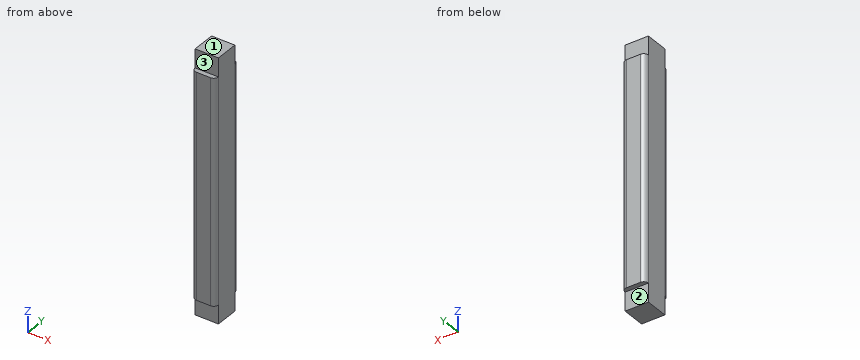
```python
from build123d import *

# Parameters (mm, degrees)
ESQUISSE1_W             = 25
ESQUISSE1_H             = 35
BOSS_EXTRU_1_DEPTH      = 280
ESQUISSE2_OUTSIDE_W     = 83.656
ESQUISSE2_OUTSIDE_H     = 93.656
ESQUISSE2_OUTSIDE_W_2   = 25
ESQUISSE2_OUTSIDE_H_2   = 25
ENL_V_MAT_EXTRU_2_DEPTH = 20
ENL_V_START             = -280
ESQUISSE2_2_OUTSIDE_W   = 83.656
ESQUISSE2_2_OUTSIDE_H   = 93.656
ESQUISSE2_2_OUTSIDE_W_2 = 25
ESQUISSE2_2_OUTSIDE_H_2 = 25
ENL_V_MAT_EXTRU_3_DEPTH = 20
CONG_1_R                = 5


with BuildPart() as part:
    # Esquisse1 → Boss.-Extru.1 (new body)
    with BuildSketch(Plane.XY):
        with Locations((12.5, 17.5)):
            Rectangle(ESQUISSE1_W, ESQUISSE1_H)
    extrude(amount=BOSS_EXTRU_1_DEPTH)

    # Esquisse2 outside → Enlèv. mat.-Extru.2 (cut)
    with BuildSketch(Plane.XY.offset(280)):
        with Locations((12.5, 17.5)):
            Rectangle(ESQUISSE2_OUTSIDE_W, ESQUISSE2_OUTSIDE_H)
        with Locations((12.5, 17.5)):
            Rectangle(ESQUISSE2_OUTSIDE_W_2, ESQUISSE2_OUTSIDE_H_2, mode=Mode.SUBTRACT)
    extrude(amount=-ENL_V_MAT_EXTRU_2_DEPTH, mode=Mode.SUBTRACT)

    # Esquisse2<2> outside → Enlèv. mat.-Extru.3 (cut)
    with BuildSketch(Plane.XY.offset(280).offset(ENL_V_START)):
        with Locations((12.5, 17.5)):
            Rectangle(ESQUISSE2_2_OUTSIDE_W, ESQUISSE2_2_OUTSIDE_H)
        with Locations((12.5, 17.5)):
            Rectangle(ESQUISSE2_2_OUTSIDE_W_2, ESQUISSE2_2_OUTSIDE_H_2, mode=Mode.SUBTRACT)
    extrude(amount=ENL_V_MAT_EXTRU_3_DEPTH, mode=Mode.SUBTRACT)

    # Congé1
    cong_1_edges = [part.edges().sort_by_distance(p)[0] for p in [
        (0, 0, 140),
        (25, 0, 140),
        (25, 35, 140),
        (0, 35, 140),
    ]]
    fillet(cong_1_edges, radius=CONG_1_R)


solid = part.part
```
Read the model definition and answer for the solid it produces. Units are mm, in the model's axes. Face numbers are marked on the shaded views. A direction names the side the tool comes from. Coordinates: 2 decimals unless noted, no trailing zeros. Order: outer loops, then holes, each group sorted by start corner. A loop starts at its lowest first (then second) coordinate and runs counter-clockwise, first axis right, second up. Notation, with made-up numbers: (1.25, 53.25) - (41.25, 53.25) arc R5 cw to (41.25, 61.25) - close; hole circle Ø6 at (73, 64). An arc over 180 degrees is marked (long way). Answer as a JSON object with one key per item and string values. Group by question number.
Item 1: Section A-A (z = 73.5) is taken. Give the vertices of the cut face in (x, y), plus the area to 3 significant figures.
Item 2: A tool of negligible diameter and unlimited length cuts with its end or side. For the marked faces 1, 2 and 3, from which of +Z, -Z, +X, -X, +Y, -Y can it reach the whole face along a straight path? Write none if from no direction.
Item 3: Flat-ended cylindrical pins translate along their axes: P1, Ø1.5, axis at x = 12.5, y = 32, coming from the +Z side; P2, Ø1.5, axis at x = 16.5, y = 1.5, coming from the -Z side; P3, Ø6, axis at x = 17, z = 272, coming from the -Y side. Find the tip coordinate at first contact, or state that the pin passes through.
Item 4: Section C-C (y = 32.5) is taken. Give the vertices of the cut face in (x, z).
Item 5: Section B-B (x = 15.25) is taken. Give the vertices of the cut face in (y, z), plus the area to 3 significant figures.
Item 6: Consider probe 1 along Z at (x, y) = (10, 33); probe 2 along Y at (x, z) = (4, 266.5); probe 3 along X at (y, z) = (33.5, 83). Determine where each line is inside the solid, lowest interval first. Write a range as from..to.
Results are:
{
 "1": {"outline": "(0, 5) arc R5 ccw to (5, 0) - (20, 0) arc R5 ccw to (25, 5) - (25, 30) arc R5 ccw to (20, 35) - (5, 35) arc R5 ccw to (0, 30) - close", "area": "854 mm^2"},
 "2": {"face 1": "+Z, +X, -X, +Y, -Y", "face 2": "-Z, +X, -X, +Y", "face 3": "+Z, +X, -X, -Y"},
 "3": {"P1": "stops at z = 260", "P2": "stops at z = 20", "P3": "stops at y = 5"},
 "4": {"outline": "(0.67, 20) - (24.33, 20) - (24.33, 260) - (0.67, 260) - close"},
 "5": {"outline": "(0, 20) - (5, 20) - (5, 0) - (30, 0) - (30, 20) - (35, 20) - (35, 260) - (30, 260) - (30, 280) - (5, 280) - (5, 260) - (0, 260) - close", "area": "9,400 mm^2"},
 "6": {"probe 1": "z = 20..260", "probe 2": "y = 5..30", "probe 3": "x = 1.43..23.57"}
}
